from build123d import *

# Parameters (mm, degrees)
F0_R     = 13
F0_R_2   = 11
F1_DEPTH = 3


with BuildPart() as f1:
    # F0 (on Front) → F1 (new body)
    with BuildSketch(Plane.XZ):
        with BuildLine():
            ThreePointArc((4.85576, 13.213033), (0, 42.40534), (-4.85576, 13.213033))
            ThreePointArc((-4.85576, 13.213033), (-4.797356, 13.193184), (-4.73887, 13.173576))
            ThreePointArc((-4.73887, 13.173576), (-4.787824, 13.155864), (-4.836711, 13.137969))
            ThreePointArc((-4.836711, 13.137969), (-12.124356, 7), (-13.79617, -2.38027))
            ThreePointArc((-13.79617, -2.38027), (-13.787224, -2.431555), (-13.778087, -2.482806))
            ThreePointArc((-13.778087, -2.482806), (-13.82431, -2.44196), (-13.870702, -2.401305))
            ThreePointArc((-13.870702, -2.401305), (-36.724102, -21.20267), (-9.014942, -10.811728))
            ThreePointArc((-9.014942, -10.811728), (-9.026955, -10.751224), (-9.039216, -10.69077))
            ThreePointArc((-9.039216, -10.69077), (-8.9994, -10.724309), (-8.95946, -10.757699))
            ThreePointArc((-8.95946, -10.757699), (0, -14), (8.95946, -10.757699))
            ThreePointArc((8.95946, -10.757699), (8.9994, -10.724309), (9.039216, -10.69077))
            ThreePointArc((9.039216, -10.69077), (9.026955, -10.751224), (9.014942, -10.811728))
            ThreePointArc((9.014942, -10.811728), (36.724102, -21.20267), (13.870702, -2.401305))
            ThreePointArc((13.870702, -2.401305), (13.82431, -2.44196), (13.778087, -2.482806))
            ThreePointArc((13.778087, -2.482806), (13.787224, -2.431555), (13.79617, -2.38027))
            ThreePointArc((13.79617, -2.38027), (12.124356, 7), (4.836711, 13.137969))
            ThreePointArc((4.836711, 13.137969), (4.787824, 13.155864), (4.73887, 13.173576))
            ThreePointArc((4.73887, 13.173576), (4.797356, 13.193184), (4.85576, 13.213033))
        make_face()
        with Locations((-23.733721, -13.70267)):
            Circle(F0_R, mode=Mode.SUBTRACT)
        with Locations((23.733721, -13.70267)):
            Circle(F0_R, mode=Mode.SUBTRACT)
        Circle(F0_R_2, mode=Mode.SUBTRACT)
        with Locations((0, 27.40534)):
            Circle(F0_R, mode=Mode.SUBTRACT)
    extrude(amount=F1_DEPTH)


solid = f1.part
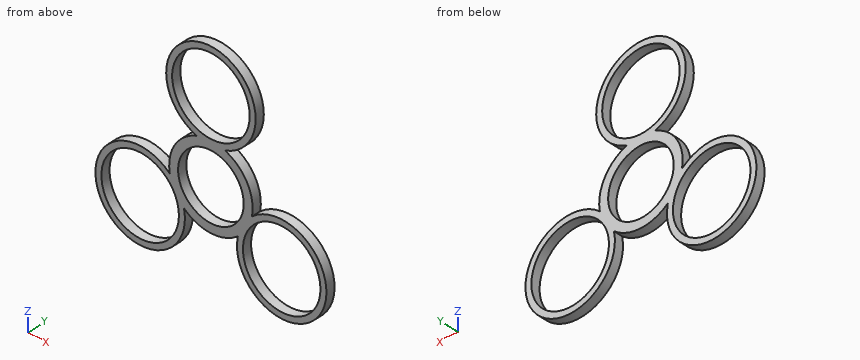
Work out the finished part from the listing and answer in its coordinate system (mm). Round coordinates to 2 decimals unless told otherwise and drop trailing zeros. Write each loop counter-clockwise with the first axis right and the second up, starting at its lowest first coordinate (ties: lowest second). Pieces come first, ordered by that corner, then holes.
1) Given pin 1 Ø1 at (y, z) = (-1, 7.5) entering from -X, flat-ended and moving along its own axis, determine where the tip first touches the part or whether it passes through.
2) A cutting plane is placed at D-D (z = -23.5). Give the vertices of the cut face in (x, y).
3) A cutting plane is placed at C-C (x = 30). Give the vertices of the cut face in (y, z), plus the area to 3 significant figures.
4) A cutting plane is placed at B-B (z = 16.5). Give the vertices of the cut face in (x, y).
5) Straight lines are drawn through the part: line 1 (X direction, y = -0.7, z = -17.5); line 2 (X direction, y = -2.3, z = 27); line 3 (Z direction, x = 24, y = -2.5). For each, find the intervals that lie inside material, in ascending order.
6) A cutting plane is placed at A-A (x = 0). Give the vertices of the cut face in (y, z).
Completed:
1. pin 1: stops at x = -12.12
2. outline: (-35.09, -3) - (-32.28, -3) - (-32.28, 0) - (-35.09, 0) - close; (-15.19, -3) - (-12.38, -3) - (-12.38, 0) - (-15.19, 0) - close; (12.38, -3) - (15.19, -3) - (15.19, 0) - (12.38, 0) - close; (32.28, -3) - (35.09, -3) - (35.09, 0) - (32.28, 0) - close
3. outline: (-3, -27.33) - (0, -27.33) - (0, -25.09) - (-3, -25.09) - close; (-3, -2.31) - (0, -2.31) - (0, -0.07) - (-3, -0.07) - close
3. area: 13.4 mm2
4. outline: (-10.3, -3) - (-7.08, -3) - (-7.08, 0) - (-10.3, 0) - close; (7.08, -3) - (10.3, -3) - (10.3, 0) - (7.08, 0) - close
5. line 1: x = -38.25 to -36.17, -11.3 to -9.22, 9.22 to 11.3, 36.17 to 38.25
5. line 2: x = -14.99 to -12.99, 12.99 to 14.99
5. line 3: z = -28.7 to -26.7, -0.71 to 1.29
6. outline: (-3, -14) - (0, -14) - (0, -11) - (-3, -11) - close; (-3, 11) - (0, 11) - (0, 14.41) - (-3, 14.41) - close; (-3, 40.41) - (0, 40.41) - (0, 42.41) - (-3, 42.41) - close
